```python
from build123d import *

# Parameters (mm, degrees)
F1_DEPTH = 25


with BuildPart() as f1:
    # F0 (on Front) → F1 (new body)
    with BuildSketch(Plane.XZ):
        with BuildLine():
            ThreePointArc((-194.281157, -111.493641), (57.693244, -216.442809), (224, 0))
            ThreePointArc((224, 0), (58.573691, 216.206204), (-193.367167, 113.071388))
            Line((-193.367167, 113.071388), (-184.133718, 107.672132))
            Line((-184.133718, 107.672132), (-176.102241, 102.975729))
            ThreePointArc((-176.102241, 102.975729), (53.343898, 196.902079), (204, 0))
            ThreePointArc((204, 0), (53.078099, -196.973895), (-176.379562, -102.5))
            ThreePointArc((-176.379562, -102.5), (-176.657747, -102.019803), (-176.934625, -101.538852))
            Line((-176.934625, -101.538852), (-187.276068, -107.473576))
            Line((-187.276068, -107.473576), (-194.281157, -111.493641))
        make_face()
        with BuildLine():
            Line((-184.133718, 107.672132), (-193.367167, 113.071388))
            ThreePointArc((-193.367167, 113.071388), (-223.998145, 0.911683), (-194.281157, -111.493641))
            Line((-194.281157, -111.493641), (-187.276068, -107.473576))
            Line((-187.276068, -107.473576), (-186.90046, -81.757066))
            ThreePointArc((-186.90046, -81.757066), (-199.67936, -41.763058), (-204, 0))
            ThreePointArc((-204, 0), (-199.048152, 44.674747), (-184.43301, 87.180645))
            Line((-184.43301, 87.180645), (-184.133718, 107.672132))
        make_face()
    extrude(amount=F1_DEPTH)


solid = f1.part
```
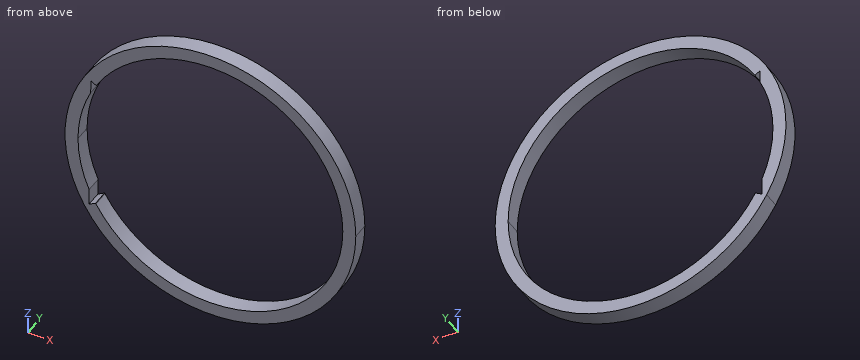
Model file for the job. Use its own axes, mm. Coordinates: 2 decimals unless noted, no trailing zeros. Order: outer loops, then holes, each group sorted by start corner. A loop starts at its lowest first (then second) coordinate and runs counter-clockwise, first axis right, second up. Notation, with made-up numbers: M 38,17 L 43,17 A18 ccw 43,49 Z; hole C 8,60 d3. An arc over 180 degrees is marked long. Answer as CSV lines item,"result".
(1) Band-saw the part on C-C, the plane x = 31. List the corners of the cut face in (y, z), then the cut area to 3 significant figures.
Geometry says:
outline,"M -25,-221.84 L 0,-221.84 L 0,-201.63 L -25,-201.63 Z; M -25,201.63 L 0,201.63 L 0,221.84 L -25,221.84 Z"
area,"1,010 mm2"
(2) Wall check: line 1 along Z through (x, y) = (-169.5, -4.25); line 2 along X through (y, z) = (-9.5, -63.5); line 3 along X through (y, z) = (-5, 175). Give the ranges that are in metal, low to high.
Geometry says:
line 1,"z = -146.44 to -113.52, 113.52 to 146.44"
line 2,"x = -214.81 to -193.87, 193.87 to 214.81"
line 3,"x = -139.82 to -104.84, 104.84 to 139.82"
(3) Flat gauge pins, fed straight in: pin 1 (3 mm diameter, centred on x = 164, y = -10.5, fed in from +Z); pin 2 (3 mm diameter, centred on y = -4, z = -35.5, fed in from -X); pin 3 (8 mm diameter, centred on x = -105, y = -7, fed in from -Z). Where does each tip first touch, or does it go through?
Geometry says:
pin 1,"stops at z = 154.17"
pin 2,"stops at x = -221.4"
pin 3,"stops at z = -199.94"
(4) Band-saw the part on A-A, the plane y = -6. List the corners of the cut face in (x, z), then the cut area to 3 significant figures.
Geometry says:
outline,"M -194.28,-111.49 A224 ccw long -193.37,113.07 A224 ccw Z; hole M -204,0 A204 ccw -186.9,-81.76 L -187.28,-107.47 L -176.93,-101.54 A204.11 ccw -176.38,-102.5 A204 ccw long -176.1,102.98 L -184.13,107.67 L -184.43,87.18 A204 ccw Z"
area,"26,700 mm2"
(5) Band-saw the part on B-B, the plane z = 134.5. List the corners of the cut face in (x, y).
Geometry says:
outline,"M -179.12,-25 L -153.38,-25 L -153.38,0 L -179.12,0 Z; M 153.38,-25 L 179.12,-25 L 179.12,0 L 153.38,0 Z"
